Autodesk Inventor part; units mm, degrees
ref_plane "YZ Plane" through (0, 0, 0) normal (1, 0, 0) x (0, 1, 0)
ref_plane "XZ Plane" through (0, 0, 0) normal (0, 1, 0) x (-1, 0, 0)
ref_plane "XY Plane" through (0, 0, 0) normal (0, 0, 1) x (1, 0, 0)
sketch "Sketch1" plane through (0, 0, 0) normal (0, 1, 0) x (-1, 0, 0)
  circle A0 centre (0, 0) radius 33
  circle A1 centre (0, 0) radius 42
  dimension "d0" = 66
  dimension "d1" = 84
extrude "Extrusion1" add sketch "Sketch1" along normal blind 18
sketch "Sketch2" plane through (0, 18, 0) normal (0, 1, 0) x (1, 0, 0)
  circle A0 centre (0, 37) radius 2
  circle A1 centre (-26.163, 26.163) radius 2
  circle A2 centre (-37, 0) radius 2
  circle A3 centre (-26.163, -26.163) radius 2
  circle A4 centre (0, -37) radius 2
  circle A5 centre (26.163, -26.163) radius 2
  circle A6 centre (37, 0) radius 2
  circle A7 centre (26.163, 26.163) radius 2
  point P0 (0, 0)
  dimension "d4" = 4
  dimension "d5" = 37
  dimension "d8" = 360
extrude "Extrusion2" cut sketch "Sketch2" against normal up to surface (18 mm away)
properties part number "Gearbox_MainBody" material "PC/ABS Plastic"
CAD build for the part. Positions are in the model's coordinates, mm. Round coordinates to 2 decimals unless told otherwise and drop trailing zeros. Write each loop counter-clockwise with the first axis right and the second up, starting at its lowest first coordinate (ties: lowest second). Pieces come first, ordered by that corner, then holes. Notation, with made-up numbers: (71, 2.25) - (127, 2.25) arc R17 cw to (127, 23.25) - close; hole circle Ø8 at (36.25, 13.5). An arc over 180 degrees is marked (long way). Return JSON: item names as keys, results as strings. Group by question number.
Item 1: Band-saw the part on C-C on z = -8. List the corners of the cut face in (x, y).
Item 2: Probe probe 1 along X at (y, z) = (13.75, 26); probe 2 along X at (y, z) = (10, -27); probe 3 along Z at (x, y) = (-25, 14). List the from-to ranges inside material, lowest first.
Item 3: Band-saw the part on A-A on x = 0. List the corners of the cut face in (y, z).
Item 4: Band-saw the part on B-B on y = 12.5. State how many separate pieces and enclosed holes the cut face has, plus the area to 3 significant figures.
Item 5: Flat gauge pins, fed straight in: pin 1 Ø6 at (x, y) = (-33, 3.5) entering from -Z; pin 2 Ø6 at (x, y) = (11.5, 12) entering from -Z; pin 3 Ø10 at (y, z) = (5.5, -31) entering from +X. Where does each tip first touch, or does it go through?
Item 6: Band-saw the part on D-D on x = -36. List the corners of the cut face in (y, z).
Item 7: Mould opens along X. For faces 1 (the face through (22, 0, -25)), 2 (the face through (0, 9, -35)), 3 (the face through (-40.06, 8.87, -12.62)) say: +X half, -X half, draft (parallel to the pull), parting line (faces both ways), or undercut.
Resolved:
{
 "1": {"outline": "(-41.23, 0) - (-32.02, 0) - (-32.02, 18) - (-41.23, 18) - close; (32.02, 0) - (41.23, 0) - (41.23, 18) - (32.02, 18) - close"},
 "2": {"probe 1": "x = -32.98 to -28.16, -24.17 to -20.32, 20.32 to 24.17, 28.16 to 32.98", "probe 2": "x = -32.17 to -27.98, -24.35 to -18.97, 18.97 to 24.35, 27.98 to 32.17", "probe 3": "z = -33.75 to -27.79, -24.54 to -21.54, 21.54 to 24.54, 27.79 to 33.75"},
 "3": {"outline": "(0, -42) - (18, -42) - (18, -39) - (0, -39) - close; (0, -35) - (18, -35) - (18, -33) - (0, -33) - close; (0, 33) - (18, 33) - (18, 35) - (0, 35) - close; (0, 39) - (18, 39) - (18, 42) - (0, 42) - close"},
 "4": {"separate pieces": "1", "enclosed holes": "9", "area": "2,020 mm²"},
 "5": {"pin 1": "stops at z = -29.39", "pin 2": "stops at z = -41.13", "pin 3": "stops at x = 32.98"},
 "6": {"outline": "(0, -21.63) - (18, -21.63) - (18, -1.73) - (0, -1.73) - close; (0, 1.73) - (18, 1.73) - (18, 21.63) - (0, 21.63) - close"},
 "7": {"face 1": "draft", "face 2": "undercut", "face 3": "parting line"}
}
